```python
from build123d import *

# Parameters (mm, degrees)
EXTRUDE_1_DEPTH     = 27.5
CUT_EXTRUDE_1_REACH = 52.806
SKETCH_4_R          = 1.5
CUT_EXTRUDE_2_REACH = 52.806
SKETCH_5_W          = 51
SKETCH_5_H          = 6.5
SKETCH_5_H_2        = 28
CUT_EXTRUDE_3_REACH = 52.806
SKETCH_6_R          = 1.375


with BuildPart() as part:
    # 草圖1 → 填料-伸長1 (new, symmetric)
    with BuildSketch(Plane.XY):
        Polygon((-25.5, 0), (-25.5, 3), (-18.5, 3), (-18.5, 13), (-40, 13), (-40, 15), (40, 15), (40, 13), (18.5, 13), (18.5, 3), (25.5, 3), (25.5, 0), (14.5, 0), (14.5, 13), (-14.5, 13), (-14.5, 0), align=None)
    extrude(amount=EXTRUDE_1_DEPTH, both=True)

    # 草圖4 → 除料-伸長1 (cut, up to next)
    with BuildSketch(Plane(origin=(0, 0, 0), x_dir=(-1, 0, 0), z_dir=(0, -1, 0)), mode=Mode.PRIVATE) as cut_extrude_1_sk1:
        with Locations(Location((-22.5, 17.5, 0), (0, 0, 90))):
            Circle(SKETCH_4_R)
    cut_extrude_1_tool1 = extrude(cut_extrude_1_sk1.sketch, amount=-CUT_EXTRUDE_1_REACH, mode=Mode.PRIVATE) & part.part
    # 草圖4 → 除料-伸長1 (cut, up to next)
    with BuildSketch(Plane(origin=(0, 0, 0), x_dir=(-1, 0, 0), z_dir=(0, -1, 0)), mode=Mode.PRIVATE) as cut_extrude_1_sk2:
        with Locations(Location((-22.5, -17.5, 0), (0, 0, 90))):
            Circle(SKETCH_4_R)
    cut_extrude_1_tool2 = extrude(cut_extrude_1_sk2.sketch, amount=-CUT_EXTRUDE_1_REACH, mode=Mode.PRIVATE) & part.part
    # 草圖4 → 除料-伸長1 (cut, up to next)
    with BuildSketch(Plane(origin=(0, 0, 0), x_dir=(-1, 0, 0), z_dir=(0, -1, 0)), mode=Mode.PRIVATE) as cut_extrude_1_sk3:
        with Locations(Location((22.5, -17.5, 0), (0, 0, 90))):
            Circle(SKETCH_4_R)
    cut_extrude_1_tool3 = extrude(cut_extrude_1_sk3.sketch, amount=-CUT_EXTRUDE_1_REACH, mode=Mode.PRIVATE) & part.part
    # 草圖4 → 除料-伸長1 (cut, up to next)
    with BuildSketch(Plane(origin=(0, 0, 0), x_dir=(-1, 0, 0), z_dir=(0, -1, 0)), mode=Mode.PRIVATE) as cut_extrude_1_sk4:
        with Locations(Location((22.5, 17.5, 0), (0, 0, 90))):
            Circle(SKETCH_4_R)
    cut_extrude_1_tool4 = extrude(cut_extrude_1_sk4.sketch, amount=-CUT_EXTRUDE_1_REACH, mode=Mode.PRIVATE) & part.part
    add(cut_extrude_1_tool1.solids().sort_by_distance((22.5, 0, -17.5))[0], mode=Mode.SUBTRACT)
    add(cut_extrude_1_tool2.solids().sort_by_distance((22.5, 0, 17.5))[0], mode=Mode.SUBTRACT)
    add(cut_extrude_1_tool3.solids().sort_by_distance((-22.5, 0, 17.5))[0], mode=Mode.SUBTRACT)
    add(cut_extrude_1_tool4.solids().sort_by_distance((-22.5, 0, -17.5))[0], mode=Mode.SUBTRACT)

    # 除料-伸長2: up to this face of the body (flat: up to its plane)
    cut_extrude_2_end = Plane(part.part.faces().sort_by_distance((0, 13, 0))[0])
    # 草圖5 → 除料-伸長2 (cut, up to the picked face)
    with BuildSketch(Plane(origin=(0, 0, 0), x_dir=(-1, 0, 0), z_dir=(0, -1, 0)), mode=Mode.PRIVATE) as cut_extrude_2_sk1:
        with Locations((0, 24.25)):
            Rectangle(SKETCH_5_W, SKETCH_5_H)
    cut_extrude_2_tool1 = split(extrude(cut_extrude_2_sk1.sketch, amount=-CUT_EXTRUDE_2_REACH, mode=Mode.PRIVATE), bisect_by=cut_extrude_2_end, keep=Keep.BOTH, mode=Mode.PRIVATE)
    # 草圖5 → 除料-伸長2 (cut, up to the picked face)
    with BuildSketch(Plane(origin=(0, 0, 0), x_dir=(-1, 0, 0), z_dir=(0, -1, 0)), mode=Mode.PRIVATE) as cut_extrude_2_sk2:
        Rectangle(SKETCH_5_W, SKETCH_5_H_2)
    cut_extrude_2_tool2 = split(extrude(cut_extrude_2_sk2.sketch, amount=-CUT_EXTRUDE_2_REACH, mode=Mode.PRIVATE), bisect_by=cut_extrude_2_end, keep=Keep.BOTH, mode=Mode.PRIVATE)
    # 草圖5 → 除料-伸長2 (cut, up to the picked face)
    with BuildSketch(Plane(origin=(0, 0, 0), x_dir=(-1, 0, 0), z_dir=(0, -1, 0)), mode=Mode.PRIVATE) as cut_extrude_2_sk3:
        with Locations((0, -24.25)):
            Rectangle(SKETCH_5_W, SKETCH_5_H)
    cut_extrude_2_tool3 = split(extrude(cut_extrude_2_sk3.sketch, amount=-CUT_EXTRUDE_2_REACH, mode=Mode.PRIVATE), bisect_by=cut_extrude_2_end, keep=Keep.BOTH, mode=Mode.PRIVATE)
    add(cut_extrude_2_tool1.solids().sort_by(Axis((0, 0, -24.25), (0, 1, 0)))[0], mode=Mode.SUBTRACT)
    add(cut_extrude_2_tool2.solids().sort_by(Axis((0, 0, 0), (0, 1, 0)))[0], mode=Mode.SUBTRACT)
    add(cut_extrude_2_tool3.solids().sort_by(Axis((0, 0, 24.25), (0, 1, 0)))[0], mode=Mode.SUBTRACT)

    # 草圖6 → 除料-伸長3 (cut, up to next)
    with BuildSketch(Plane(origin=(0, 15, 0), x_dir=(1, 0, 0), z_dir=(0, 1, 0)), mode=Mode.PRIVATE) as cut_extrude_3_sk1:
        with Locations(Location((-35, 24.5, 0), (0, 0, 270))):
            Circle(SKETCH_6_R)
    cut_extrude_3_tool1 = extrude(cut_extrude_3_sk1.sketch, amount=-CUT_EXTRUDE_3_REACH, mode=Mode.PRIVATE) & part.part
    # 草圖6 → 除料-伸長3 (cut, up to next)
    with BuildSketch(Plane(origin=(0, 15, 0), x_dir=(1, 0, 0), z_dir=(0, 1, 0)), mode=Mode.PRIVATE) as cut_extrude_3_sk2:
        with Locations(Location((-35, -24.5, 0), (0, 0, 270))):
            Circle(SKETCH_6_R)
    cut_extrude_3_tool2 = extrude(cut_extrude_3_sk2.sketch, amount=-CUT_EXTRUDE_3_REACH, mode=Mode.PRIVATE) & part.part
    # 草圖6 → 除料-伸長3 (cut, up to next)
    with BuildSketch(Plane(origin=(0, 15, 0), x_dir=(1, 0, 0), z_dir=(0, 1, 0)), mode=Mode.PRIVATE) as cut_extrude_3_sk3:
        with Locations(Location((23, -24.5, 0), (0, 0, 270))):
            Circle(SKETCH_6_R)
    cut_extrude_3_tool3 = extrude(cut_extrude_3_sk3.sketch, amount=-CUT_EXTRUDE_3_REACH, mode=Mode.PRIVATE) & part.part
    # 草圖6 → 除料-伸長3 (cut, up to next)
    with BuildSketch(Plane(origin=(0, 15, 0), x_dir=(1, 0, 0), z_dir=(0, 1, 0)), mode=Mode.PRIVATE) as cut_extrude_3_sk4:
        with Locations(Location((23, 24.5, 0), (0, 0, 270))):
            Circle(SKETCH_6_R)
    cut_extrude_3_tool4 = extrude(cut_extrude_3_sk4.sketch, amount=-CUT_EXTRUDE_3_REACH, mode=Mode.PRIVATE) & part.part
    add(cut_extrude_3_tool1.solids().sort_by_distance((-35, 15, -24.5))[0], mode=Mode.SUBTRACT)
    add(cut_extrude_3_tool2.solids().sort_by_distance((-35, 15, 24.5))[0], mode=Mode.SUBTRACT)
    add(cut_extrude_3_tool3.solids().sort_by_distance((23, 15, 24.5))[0], mode=Mode.SUBTRACT)
    add(cut_extrude_3_tool4.solids().sort_by_distance((23, 15, -24.5))[0], mode=Mode.SUBTRACT)


solid = part.part
```
Check sheet for the modelled part. Datum: model origin and axes. Units: mm. A direction names the side the tool comes from. Round coordinates to 2 decimals unless told otherwise and drop trailing zeros. Loops run counter-clockwise (first coordinate to the right, second up) from the corner with the lowest first, then second, coordinate; pieces in that order, holes last. Notation, with made-up numbers: (1.5, -8) - (14.5, -8) arc R31 ccw to (14.5, 18) - close; hole circle Ø10 at (70.5, -20). An arc over 180 degrees is marked (long way). Answer as a JSON object with one key per item and string values. Group by question number.
Q1. Set-up check for faces 1 (the face through (-14.5, 7, -17)), 2 (the face through (23.51, 1.48, 18.61)), 3 (the face through (18, 5, -14)): record each of +Z, -Z, +X, -X, +Y, -Y from which the full face is reachable in a straight line by a thin tool's end or side.
Q2. Gauge pin test, flat ends, axial feed: P1, Ø3.5, axis at y = 7, z = 16.5, coming from the -X side; P2, Ø2.5, axis at y = 1, z = -19, coming from the +X side; P3, Ø5.5, axis at x = -19.5, y = 8, coming from the +Z side. Record the tip position at first contact, or that the pin passes through.
Q3. Scan lines: line 1 along X through (y, z) = (14.2, -24.5) (3 decimals); line 2 along X through (y, z) = (0.5, 20.5); line 3 along Y through (x, z) = (30.5, 1.5). Record each from-to range of solid material in increasing order. Write a range as [from, to].
Q4. Sectioned sample at A-A, the plane z = -24.5. Enter the section's corners in (x, y) (3 decimals).
Q5. Sectioned sample at B-B, the plane x = -35. Enter the section's corners in (y, z) (3 decimals).
Q6. Sectioned sample at D-D, the plane x = -22.5. Enter the section's corners in (y, z), plus the area to 3 significant figures.
Q7. Mould release check, pull along Y, two halves, no side actions. Record for faces 4 (the face through (20, 3, 18)), 5 (the face through (23.929, 14.014, 23.487)), 6 (the face through (-20, 0, 18)): released by +Y, released by -Y, zero draft, split by the parting line, or undercut.
Q8. Sectioned sample at C-C, the plane y = 2. Enter the section's corners in (x, z), plus the area to 3 significant figures.
Solution:
{
 "1": {"face 1": "+Z, -Z, -Y", "face 2": "-Y", "face 3": "+X, -X, -Y"},
 "2": {"P1": "stops at x = -18.5", "P2": "stops at x = 25.5", "P3": "stops at z = 21"},
 "3": {"line 1": "x = [-40, -36.375], [-33.625, 21.625], [24.375, 40]", "line 2": "x = [-25.5, -14.5], [14.5, 25.5]", "line 3": "y = [13, 15]"},
 "4": {"outline": "(-40, 13) - (-36.375, 13) - (-36.375, 15) - (-40, 15) - close; (-33.625, 13) - (21.625, 13) - (21.625, 15) - (-33.625, 15) - close; (24.375, 13) - (40, 13) - (40, 15) - (24.375, 15) - close"},
 "5": {"outline": "(13, -27.5) - (15, -27.5) - (15, -25.875) - (13, -25.875) - close; (13, -23.125) - (15, -23.125) - (15, 23.125) - (13, 23.125) - close; (13, 25.875) - (15, 25.875) - (15, 27.5) - (13, 27.5) - close"},
 "6": {"outline": "(0, -21) - (3, -21) - (3, -19) - (0, -19) - close; (0, -16) - (3, -16) - (3, -14) - (0, -14) - close; (0, 14) - (3, 14) - (3, 16) - (0, 16) - close; (0, 19) - (3, 19) - (3, 21) - (0, 21) - close; (13, -27.5) - (15, -27.5) - (15, 27.5) - (13, 27.5) - close", "area": "134 mm²"},
 "7": {"face 4": "undercut", "face 5": "zero draft", "face 6": "released by -Y"},
 "8": {"outline": "(-25.5, -21) - (-14.5, -21) - (-14.5, -14) - (-25.5, -14) - close; (-25.5, 14) - (-14.5, 14) - (-14.5, 21) - (-25.5, 21) - close; (14.5, -21) - (25.5, -21) - (25.5, -14) - (14.5, -14) - close; (14.5, 14) - (25.5, 14) - (25.5, 21) - (14.5, 21) - close; hole circle Ø3 at (-22.5, -17.5); hole circle Ø3 at (-22.5, 17.5); hole circle Ø3 at (22.5, -17.5); hole circle Ø3 at (22.5, 17.5)", "area": "280 mm²"}
}
